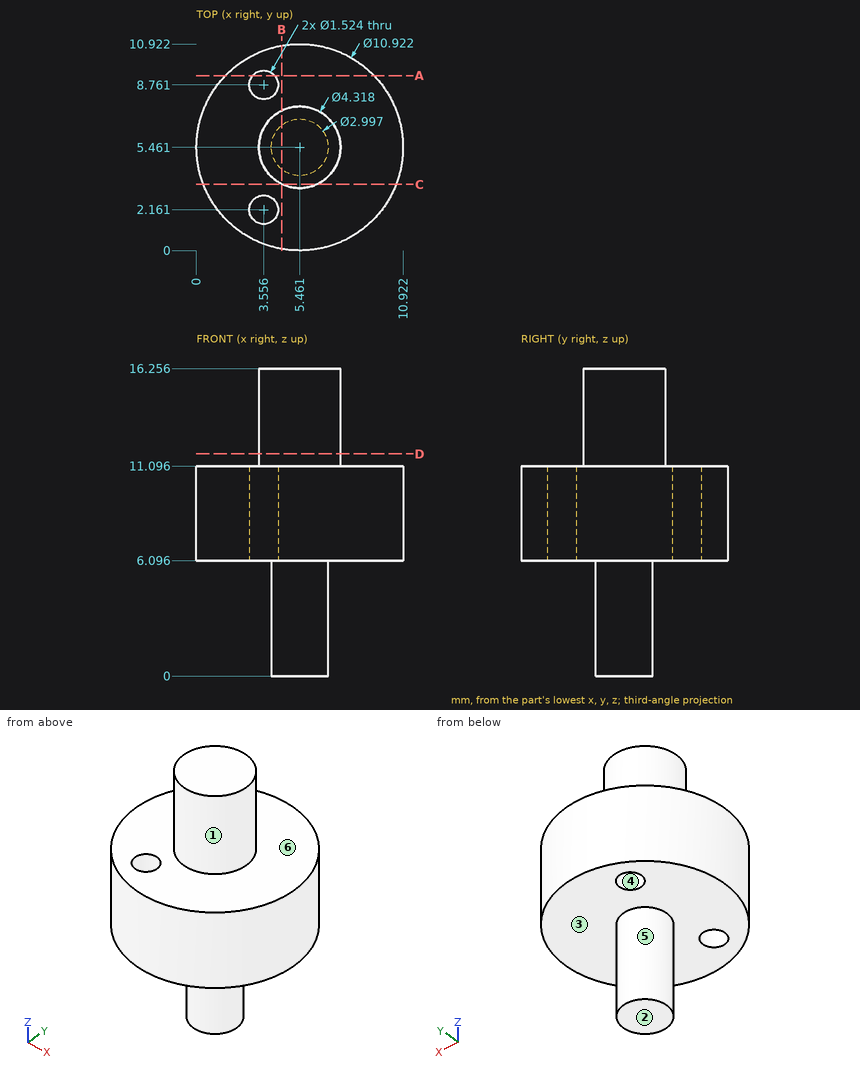
Job drawing, mm, ordinate dimensions from the low corner. One solid piece. A direction names the side the tool comes from. Coordinates: 2 decimals unless noted, no trailing zeros. Write each loop counter-clockwise with the first axis right and the second up, starting at its lowest first coordinate (ties: lowest second). Pieces come first, ordered by that corner, then holes. Notation, with made-up numbers: (0.5, 0) - (27.5, 0) arc R17 ccw to (27.5, 12) - close; hole circle Ø7 at (-21.5, -36). An arc over 180 degrees is marked (long way). Use a Markdown table: item, result. Add a question column.
Item 1: Drill centre lines: L1, parallel to Y at x = 3.75, z = 10.25 (1 decimal); L2, parallel to Y at x = 3.25, z = 6.75 (1 decimal); L3, parallel to Z at x = 10, y = 4.75. Where is each one in solid material? Low to high. Write a range as from..to.
Item 2: Band-saw the part on C-C, the plane y = 3.5. Give the cut face in (x, z) (1 decimal).
Item 3: 3-axis set-ups, long thin cutter, end or side, ignore diameter. For the marked faces 1, 2 and 3: which of +Z, -Z, +X, -X, +Y, -Y reach the whole face in a straight line?
Item 4: Band-saw the part on A-A, the plane y = 9.25. Give the cut face in (x, z).
Item 5: Band-saw the part on D-D, the plane z = 11.75. Give the cut face in (x, y).
Item 6: Flat gauge pins, fed straight in: pin 1 (6 mm diameter, centred on x = 5, z = 2, fed in from -Y); pin 2 (1 mm diameter, centred on y = 9, z = 10, fed in from +X); pin 3 (1 mm diameter, centred on x = 6, y = 8.5, fed in from +Z). Where does each tip first touch, or does it go through?
Item 7: Mould opens along X. For the marked faces 4, 5 and 6 say: pulls with the +X half, pulls with the -X half, needs draft (parallel to the pull), parting line crosses it, or undercut.
Item 8: Band-saw the part on B-B, the plane x = 4.5. Give the cut face in (y, z) (1 decimal).
Numbers:
| question | item | result |
|---|---|---|
| 1 | L1 | 0.3..1.4, 2.9..8, 9.5..10.6 |
| 1 | L2 | 0.5..1.5, 2.9..8.1, 9.5..10.5 |
| 1 | L3 | 6.1..11.1 |
| 2 | outline | (0.4, 6.1) - (10.6, 6.1) - (10.6, 11.1) - (6.4, 11.1) - (6.4, 16.3) - (4.6, 16.3) - (4.6, 11.1) - (0.4, 11.1) - close |
| 3 | face 1 | +Z |
| 3 | face 2 | -Z, +X, -X, +Y, -Y |
| 3 | face 3 | -Z |
| 4 | outline | (1.53, 6.1) - (2.97, 6.1) - (2.97, 11.1) - (1.53, 11.1) - close; (4.14, 6.1) - (9.39, 6.1) - (9.39, 11.1) - (4.14, 11.1) - close |
| 5 | outline | circle Ø4.32 at (5.46, 5.46) |
| 6 | pin 1 | y = 3.96 |
| 6 | pin 2 | x = 10 |
| 6 | pin 3 | z = 11.1 |
| 7 | face 4 | undercut |
| 7 | face 5 | parting line crosses it |
| 7 | face 6 | needs draft |
| 8 | outline | (0.1, 6.1) - (4.3, 6.1) - (4.3, 0) - (6.6, 0) - (6.6, 6.1) - (10.8, 6.1) - (10.8, 11.1) - (7.4, 11.1) - (7.4, 16.3) - (3.5, 16.3) - (3.5, 11.1) - (0.1, 11.1) - close |
